Autodesk Fusion 360 part; units mm, degrees
sketch "Sketch1" plane through (0, 0, 0) normal (0, 0, 1) x (1, 0, 0)
  circle A0 centre (0, 0) radius 12.5
  dimension "d1" = 25
extrude "Extrude1" add sketch "Sketch1" along normal blind 37 draft 5
shell "Shell1" thickness 1 removed faces 1 at (-7.81, 2.0449, 37)
fillet "Fillet1" radius 0.5 2 edges at (-14.6721, 5.6908, 37) (-13.7362, 5.3278, 37)
fillet "Fillet2" radius 0.5 1 edges at (-11.6541, -4.5202, 0)
Design review of the part built by this model. Coordinates are the model's own, in mm. Coordinates: 2 decimals unless noted, no trailing zeros. Order: outer loops, then holes, each group sorted by start corner. A loop starts at its lowest first (then second) coordinate and runs counter-clockwise, first axis right, second up. Notation, with made-up numbers: (-31.5, -8.75) -> (20.5, -8.75) arc R11 ccw to (20.5, -2.75) -> close; hole circle Ø6 at (48, 65). An arc over 180 degrees is marked (long way). One line per item, written item: value. Start each with the question number.
Q1. Take a section at C-C, the plane z = 17. State the section outline as (x, y) points, then the cut area to 3 significant figures.
Q2. Insertion check: pin 1 Ø4 at (y, z) = (0.5, 19.5) entering from -X; pin 2 Ø4 at (x, z) = (-8, 13.5) entering from +Y; pin 3 Ø8 at (x, z) = (-7.5, 12) entering from +Y; pin 4 Ø1 at (x, y) = (3.5, -6) entering from -Z. Each pin has a flat end and moves straight along its axis. Give the tip position at first contact, or say it passes through.
Q3. Take a section at D-D, the plane z = 6. State the section outline as (x, y) points, then the cut area to 3 significant figures.
Q4. For probe 1 along Z at (x, y) = (-8, 3); probe 2 along X at (y, z) = (6.5, 33); probe 3 along Y at (x, z) = (-9, 20.5), list the stretches that pass through material, from the lowest coordinate up.
Q5. Mouldability with a two-part tool opening along X and no side actions: class faces 1 (the flat face through (0, 0, 0)), 2 (the conical face through (-3.06, -13.8, 18.71)), 3 (the flat face through (0, 0, 1)) as pulls with the +X half, pulls with the -X half, needs draft (parallel to the pull), parting line crosses it, or undercut.
Values follow:
1. outline: circle Ø27.97 at (0, 0); hole circle Ø25.97 at (0, 0)
1. area: 85.1 mm2
2. pin 1: stops at x = -14.38
2. pin 2: stops at y = 12.31
2. pin 3: stops at y = 13.15
2. pin 4: stops at z = 0
3. outline: circle Ø26.05 at (0, 0); hole circle Ø24.04 at (0, 0)
3. area: 79.0 mm2
4. probe 1: z = 0 to 1
4. probe 2: x = -13.95 to -12.83, 12.83 to 13.95
4. probe 3: y = -11.1 to -9.78, 9.78 to 11.1
5. face 1: needs draft
5. face 2: parting line crosses it
5. face 3: undercut
